from build123d import *

# Parameters (mm, degrees)
SKETCH_1_R          = 7.5
SKETCH_1_R_2        = 4
EXTRUDE_1_DEPTH     = 5
CHAMFER_1_SIZE      = 0.5
CHAMFER_2_SIZE      = 0.5
SKETCH_2_R          = 6.5
SKETCH_2_R_2        = 4.75
CUT_EXTRUDE_1_DEPTH = 0.8
CUT_EXTRUDE_START   = -0.8
SKETCH_3_R          = 6.5
SKETCH_3_R_2        = 4.75
CUT_EXTRUDE_2_DEPTH = 0.8


with BuildPart() as part:
    # 草图1 → 凸台-拉伸1 (new body)
    with BuildSketch(Plane(origin=(0, 0, 0), x_dir=(1, 0, 0), z_dir=(0, 1, 0))):
        with Locations(Location((0, 0, 0), (0, 0, 270))):
            Circle(SKETCH_1_R)
        with Locations(Location((0, 0, 0), (0, 0, 270))):
            Circle(SKETCH_1_R_2, mode=Mode.SUBTRACT)
    extrude(amount=EXTRUDE_1_DEPTH)

    # 倒角1
    chamfer_1_edges = [part.edges().sort_by_distance(p)[0] for p in [
        (0, 5, -7.5),
    ]]
    chamfer(chamfer_1_edges, length=CHAMFER_1_SIZE)

    # 倒角2
    chamfer_2_edges = [part.edges().sort_by_distance(p)[0] for p in [
        (0, 0, -7.5),
    ]]
    chamfer(chamfer_2_edges, length=CHAMFER_2_SIZE)

    # 草图2 → 切除-拉伸1 (cut)
    with BuildSketch(Plane(origin=(0, 5, 0), x_dir=(1, 0, 0), z_dir=(0, 1, 0))):
        with Locations(Location((0, 0, 0), (0, 0, 270))):
            Circle(SKETCH_2_R)
        with Locations(Location((0, 0, 0), (0, 0, 270))):
            Circle(SKETCH_2_R_2, mode=Mode.SUBTRACT)
    extrude(amount=-CUT_EXTRUDE_1_DEPTH, mode=Mode.SUBTRACT)

    # 草图3 → 切除-拉伸2 (cut)
    with BuildSketch(Plane.XZ.offset(CUT_EXTRUDE_START)):
        with Locations(Location((0, 0, 0), (0, 0, 90))):
            Circle(SKETCH_3_R)
        with Locations(Location((0, 0, 0), (0, 0, 90))):
            Circle(SKETCH_3_R_2, mode=Mode.SUBTRACT)
    extrude(amount=CUT_EXTRUDE_2_DEPTH, mode=Mode.SUBTRACT)


solid = part.part
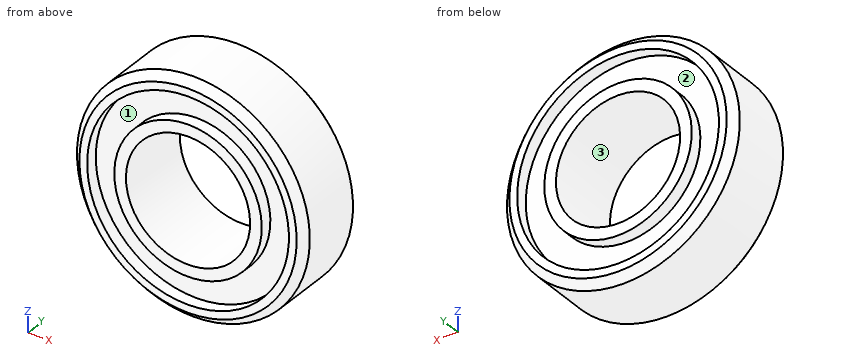
Geometry check sheet. Reference: the model listing, model coordinates, mm. Face numbers are marked on the shaded views. A direction names the side the tool comes from. Round coordinates to 2 decimals unless told otherwise and drop trailing zeros. Loops run counter-clockwise (first coordinate to the right, second up) from the corner with the lowest first, then second, coordinate; pieces in that order, holes last. Notation, with made-up numbers: (68, -17) - (74, -17) arc R16 cw to (74, 4) - close; hole circle Ø6 at (-26.5, 18). An arc over 180 degrees is marked (long way). Answer as CSV lines item,"result".
(1) Set-up check for the marked faces 1, 2 and 3: record each of +Z, -Z, +X, -X, +Y, -Y from which the full face is reachable in a straight line by a thin tool's end or side.
Output values:
face 1,"-Y"
face 2,"+Y"
face 3,"+Y, -Y"
(2) Cross-section at C-C, the plane y = 3.1. Enter the section's corners in (x, z), and give its area (3 significant figures).
Output values:
outline,"circle Ø15 at (0, 0); hole circle Ø8 at (0, 0)"
area,"126 mm²"
(3) Cross-section at B-B, the plane z = 0. Enter the section's corners in (x, y).
Output values:
outline,"(-7.5, 0.5) - (-7, 0) - (-6.5, 0) - (-6.5, 0.8) - (-4.75, 0.8) - (-4.75, 0) - (-4, 0) - (-4, 5) - (-4.75, 5) - (-4.75, 4.2) - (-6.5, 4.2) - (-6.5, 5) - (-7, 5) - (-7.5, 4.5) - close; (4, 0) - (4.75, 0) - (4.75, 0.8) - (6.5, 0.8) - (6.5, 0) - (7, 0) - (7.5, 0.5) - (7.5, 4.5) - (7, 5) - (6.5, 5) - (6.5, 4.2) - (4.75, 4.2) - (4.75, 5) - (4, 5) - close"
(4) Material ranges on line 1 along X through (y, z) = (0.6, 0); line 2 along X through (y, z) = (2.7, 0); line 3 along X through (y, z) = (0.3, 0), recorded low to high.
Output values:
line 1,"x = -7.5 to -6.5, -4.75 to -4, 4 to 4.75, 6.5 to 7.5"
line 2,"x = -7.5 to -4, 4 to 7.5"
line 3,"x = -7.3 to -6.5, -4.75 to -4, 4 to 4.75, 6.5 to 7.3"
(5) Cross-section at A-A, the plane x = 0. Enter the section's corners in (y, z), and give its area (3 significant figures).
Output values:
outline,"(0, -7) - (0.5, -7.5) - (4.5, -7.5) - (5, -7) - (5, -6.5) - (4.2, -6.5) - (4.2, -4.75) - (5, -4.75) - (5, -4) - (0, -4) - (0, -4.75) - (0.8, -4.75) - (0.8, -6.5) - (0, -6.5) - close; (0, 4) - (5, 4) - (5, 4.75) - (4.2, 4.75) - (4.2, 6.5) - (5, 6.5) - (5, 7) - (4.5, 7.5) - (0.5, 7.5) - (0, 7) - (0, 6.5) - (0.8, 6.5) - (0.8, 4.75) - (0, 4.75) - close"
area,"28.9 mm²"
(6) Depth check by flat-ended pin: pin 1 Ø1 at (x, y) = (-5.5, 3) entering from +Z; pin 2 Ø3 at (x, y) = (3, 4) entering from -Z; pin 3 Ø7 at (x, z) = (0, 0) entering from +Y. Enter the tip coordinate at first touch or a pass-through.
Output values:
pin 1,"stops at z = 5.59"
pin 2,"stops at z = -7.35"
pin 3,"passes through"
